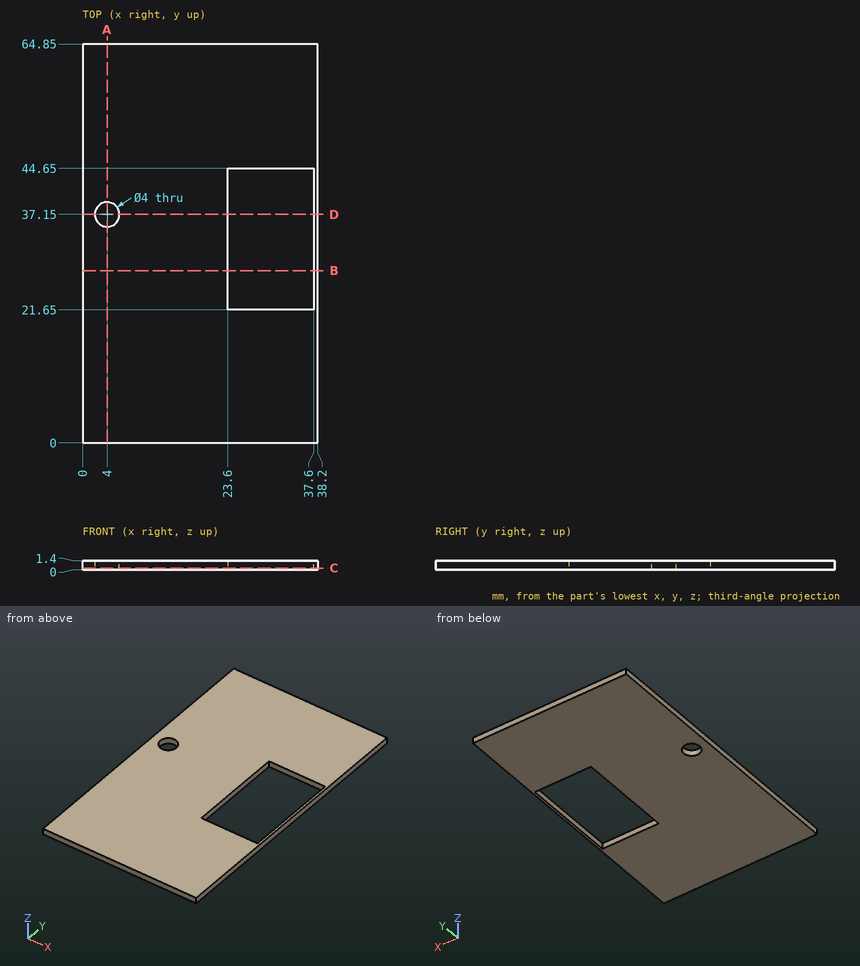
Here's the drawing with two shaded views (mm, measured from the low corner). I have some questions. Round coordinates to 2 decimals unless told otherwise and drop trailing zeros. Write each loop counter-clockwise with the first axis right and the second up, starting at its lowest first coordinate (ties: lowest second). Pieces come first, ordered by that corner, then holes. Notation, with made-up numbers: M 80,82 L 122,82 A25 ccw 122,96 Z; hole C 45,55 d7. An arc over 180 degrees is marked long. Answer in a Markdown table with one row per item. Add a question column.
Q1. If I drill on line 1 (X direction, y = 37.15, z = 0.75); line 2 (Y direction, x = 4, z = 0.65); line 3 (Y direction, x = 27.5, z = 1), over which ranges is the centre line in solid material (lowest first)? Write a range as from..to.
Q2. Will this pin go through, and if not, where does the flat tip stop? pin 1 Ø2 at (x, y) = (8.5, 28.5) entering from -Z.
Q3. Imagine slicing it at D-D (y = 37.15). Please give me the cut outline in (x, z), then the cut area to 3 significant figures.
Q4. Imagine slicing it at A-A (x = 4). Please give me the cut outline in (y, z), then the cut area to 3 significant figures.
Q5. Imagine slicing it at C-C (z = 0.25). Please give me the cut outline in (x, y), then the cut area to 3 significant figures.
Q6. Imagine slicing it at B-B (y = 28). Please give me the cut outline in (x, z).
Values:
| question | item | result |
|---|---|---|
| 1 | line 1 | 0..2, 6..23.6, 37.6..38.2 |
| 1 | line 2 | 0..35.15, 39.15..64.85 |
| 1 | line 3 | 0..21.65, 44.65..64.85 |
| 2 | pin 1 | z = 0 |
| 3 | outline | M 0,0 L 2,0 L 2,1.4 L 0,1.4 Z; M 6,0 L 23.6,0 L 23.6,1.4 L 6,1.4 Z; M 37.6,0 L 38.2,0 L 38.2,1.4 L 37.6,1.4 Z |
| 3 | area | 28.3 mm^2 |
| 4 | outline | M 0,0 L 35.15,0 L 35.15,1.4 L 0,1.4 Z; M 39.15,0 L 64.85,0 L 64.85,1.4 L 39.15,1.4 Z |
| 4 | area | 85.2 mm^2 |
| 5 | outline | M 0,0 L 38.2,0 L 38.2,64.85 L 0,64.85 Z; hole C 4,37.15 d4; hole M 23.6,21.65 L 37.6,21.65 L 37.6,44.65 L 23.6,44.65 Z |
| 5 | area | 2,140 mm^2 |
| 6 | outline | M 0,0 L 23.6,0 L 23.6,1.4 L 0,1.4 Z; M 37.6,0 L 38.2,0 L 38.2,1.4 L 37.6,1.4 Z |
